Here's the drawing with two shaded views (mm, measured from the low corner). I have some questions. Give positions to 0.01 mm unless a question says otherwise; leave off trailing zeros. Write each loop counter-clockwise with the first axis right and the second up, starting at its lowest first coordinate (ties: lowest second). Pieces come first, ordered by that corner, then holes.
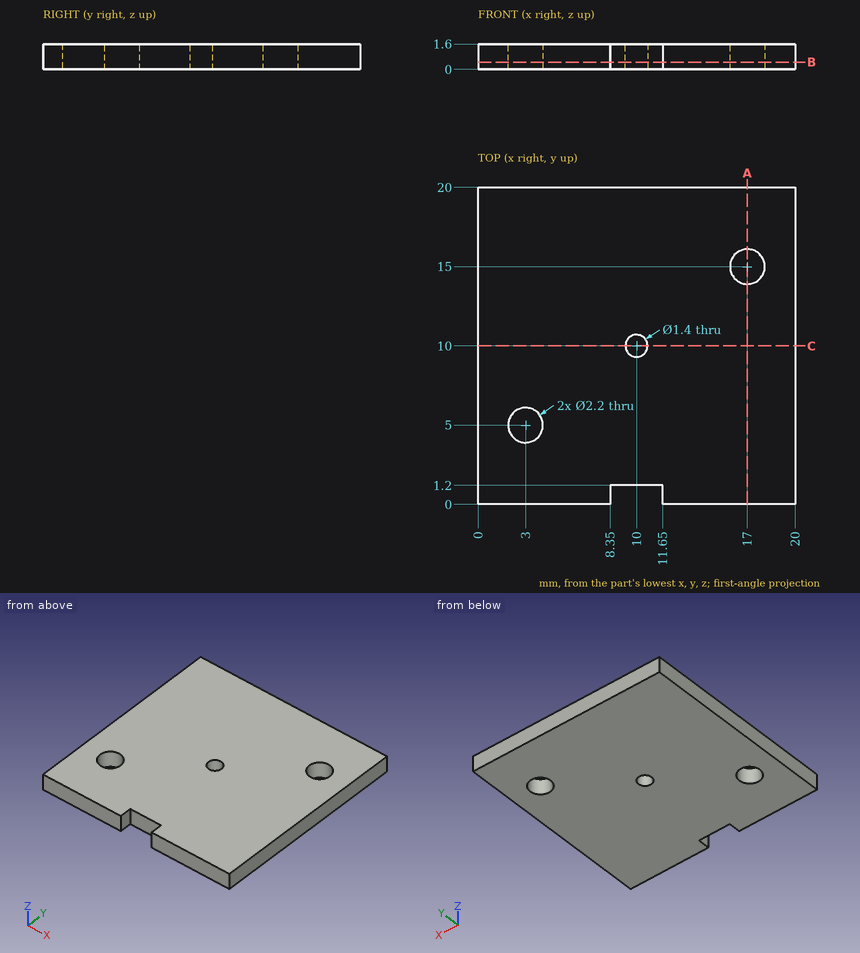
(1) Imagine slicing it at B-B, the plane z = 0.45. Write out the boundary of the cut face in (x, y).
Returned:
outline: (0, 0) - (8.35, 0) - (8.35, 1.2) - (11.65, 1.2) - (11.65, 0) - (20, 0) - (20, 20) - (0, 20) - close; hole circle Ø2.2 at (3, 5); hole circle Ø1.4 at (10, 10); hole circle Ø2.2 at (17, 15)
(2) Imagine slicing it at C-C, the plane y = 10. Write out the boundary of the cut face in (x, z), plus the area to 3 significant figures.
Returned:
outline: (0, 0) - (9.3, 0) - (9.3, 1.6) - (0, 1.6) - close; (10.7, 0) - (20, 0) - (20, 1.6) - (10.7, 1.6) - close
area: 29.8 mm2
(3) Will this pin go through, and if not, where does the flat tip stop? P1, Ø12, axis at x = 7, y = 7, coming from the -Z side.
Returned:
P1: stops at z = 0
(4) If I drill on L1, parallel to Y at x = 3, z = 1.05; L2, parallel to Y at x = 17, z = 0.55; L3, parallel to X at y = 4.25, z = 0.4, over which ranges is the centre line in solid material (lowest first)?
Returned:
L1: y = 0 to 3.9, 6.1 to 20
L2: y = 0 to 13.9, 16.1 to 20
L3: x = 0 to 2.2, 3.8 to 20
(5) Imagine slicing it at A-A, the plane x = 17. Write out the boundary of the cut face in (y, z), plus the area to 3 significant figures.
Returned:
outline: (0, 0) - (13.9, 0) - (13.9, 1.6) - (0, 1.6) - close; (16.1, 0) - (20, 0) - (20, 1.6) - (16.1, 1.6) - close
area: 28.5 mm2
